Autodesk Inventor part; units mm, degrees
ref_plane "YZ Plane" through (0, 0, 0) normal (1, 0, 0) x (0, 1, 0)
ref_plane "XZ Plane" through (0, 0, 0) normal (0, 1, 0) x (-1, 0, 0)
ref_plane "XY Plane" through (0, 0, 0) normal (0, 0, 1) x (1, 0, 0)
sketch "Sketch1" plane through (0, 0, 0) normal (0, 0, 1) x (1, 0, 0)
  line L0 (-35.5, 13.25) -> (35.5, 13.25)
  line L1 (35.5, 13.25) -> (35.5, -13.25)
  line L2 (35.5, -13.25) -> (-35.5, -13.25)
  line L3 (-35.5, -13.25) -> (-35.5, 13.25)
  line L4 (-34.3, 12.05) -> (34.3, 12.05)
  line L5 (34.3, 12.05) -> (34.3, -12.05)
  line L6 (34.3, -12.05) -> (-34.3, -12.05)
  line L7 (-34.3, -12.05) -> (-34.3, 12.05)
  point P0 (0, 0)
  dimension "d0" = 71
  dimension "d1" = 26.5
  dimension "d2" = 35.5
  dimension "d3" = 13.25
  dimension "d4" = 1.2
  dimension "d5" = 1.2
  dimension "d6" = 1.2
  dimension "d7" = 1.2
extrude "Extrusion1" add sketch "Sketch1" along normal blind 100
fillet "Fillet1" radius 2 4 edges at (-34.3, 12.05, 50) (34.3, 12.05, 50) (34.3, -12.05, 50) (-34.3, -12.05, 50)
fillet "Fillet2" radius 3.25 4 edges at (-35.5, 13.25, 50) (-35.5, -13.25, 50) (35.5, -13.25, 50) (35.5, 13.25, 50)
sketch "Sketch2" plane through (0, 0, 100) normal (0, 0, 1) x (1, 0, 0)
  line L0 (-34.3, -10.05) -> (-34.3, 10.05)
  line L1 (-34.3, -7.9) -> (-31.3, -7.9)
  line L2 (-31.3, -7.9) -> (-31.3, -9.4)
  line L3 (-31.3, -9.4) -> (-34.3, -9.4)
  line L4 (-34.3, -9.4) -> (-34.3, -7.9)
  line L5 (34.3, 10.05) -> (34.3, -10.05)
  line L6 (34.3, -7.9) -> (31.3, -7.9)
  line L7 (31.3, -7.9) -> (31.3, -9.4)
  line L8 (31.3, -9.4) -> (34.3, -9.4)
  line L9 (34.3, -9.4) -> (34.3, -7.9)
  line L10 (-32.25, -13.25) -> (32.25, -13.25)
  line L11 (-34.3, -5.9) -> (-31.3, -5.9)
  line L12 (-31.3, -5.9) -> (-31.3, -4.4)
  line L13 (-31.3, -4.4) -> (-34.3, -4.4)
  line L14 (-34.3, -4.4) -> (-34.3, -5.9)
  line L15 (31.3, -5.9) -> (34.3, -5.9)
  line L16 (34.3, -5.9) -> (34.3, -4.4)
  line L17 (34.3, -4.4) -> (31.3, -4.4)
  line L18 (31.3, -4.4) -> (31.3, -5.9)
  point P0 (0, 0)
  dimension "d12" = 3.85
  dimension "d13" = 1.5
  dimension "d14" = 3
  dimension "d15" = 3
  dimension "d16" = 1.5
  dimension "d17" = 2
extrude "Extrusion2" add sketch "Sketch2" against normal blind 100
fillet "Fillet3" radius 1 4 edges at (-34.3, -4.4, 50) (-34.3, -9.4, 50) (34.3, -9.4, 50) (34.3, -4.4, 50)
sketch "Sketch3" plane through (0, 0, 100) normal (0, 0, 1) x (1, 0, 0)
  line L0 (32.25, 13.25) -> (-32.25, 13.25)
  line L1 (-35.5, 10) -> (-35.5, -10)
  line L2 (-32.25, -13.25) -> (32.25, -13.25)
  line L3 (35.5, -10) -> (35.5, 10)
  circle A0 centre (-32.5, 10.25) radius 2.25
  circle A1 centre (-32.5, -10.25) radius 2.25
  circle A2 centre (32.5, -10.25) radius 2.25
  circle A3 centre (32.5, 10.25) radius 2.25
  point P0 (0, 0)
  dimension "d21" = 3
  dimension "d22" = 3
  dimension "d23" = 3
  dimension "d24" = 3
  dimension "d25" = 3
  dimension "d26" = 3
  dimension "d27" = 3
  dimension "d28" = 3
  dimension "d29" = 4.5
  dimension "d30" = 4.5
  dimension "d31" = 4.5
  dimension "d32" = 4.5
extrude "Extrusion3" add sketch "Sketch3" against normal blind 100
sketch "Sketch4" plane through (0, 0, 100) normal (0, 0, 1) x (1, 0, 0)
  arc A0 (-34.3, 8.9) -> (-31.15, 12.05) centre (-32.5, 10.25) ccw
  arc A1 (31.15, 12.05) -> (34.3, 8.9) centre (32.5, 10.25) ccw
  arc A2 (31.3, -8.3467) -> (31.15, -12.05) centre (32.5, -10.25) ccw
  arc A3 (-31.15, -12.05) -> (-31.3, -8.3467) centre (-32.5, -10.25) ccw
  circle A4 centre (-32.5, 10.25) radius 1.25
  circle A5 centre (-32.5, -10.25) radius 1.25
  circle A6 centre (32.5, 10.25) radius 1.25
  circle A7 centre (32.5, -10.25) radius 1.25
  point P0 (0, 0)
  dimension "d35" = 2.5
  dimension "d36" = 2.5
  dimension "d37" = 2.5
  dimension "d38" = 2.5
extrude "Extrusion4" cut sketch "Sketch4" against normal blind 100
sketch "Sketch6" plane through (0, 0, 100) normal (0, 0, 1) x (1, 0, 0)
  line L0 (34.3, -5.9) -> (34.3, -7.9)
  line L1 (-34.3, -7.9) -> (-34.3, -5.9)
  line L2 (-31.3, -7.9) -> (-34.3, -7.9)
  line L3 (-31.3, -7.9) -> (-31.5, -7.9)
  line L4 (-31.5, -7.9) -> (-31.5, -9.4)
  line L5 (-31.5, -9.4) -> (-31.3, -9.4)
  line L6 (-31.3, -9.4) -> (-31.3, -7.9)
  line L7 (-31.3, -5.9) -> (-31.3, -4.4)
  line L8 (-31.3, -4.4) -> (-31.5, -4.4)
  line L9 (-31.5, -4.4) -> (-31.5, -5.9)
  line L10 (-31.5, -5.9) -> (-31.3, -5.9)
  line L11 (-31.3, -5.9) -> (-31.3, -4.4)
  line L12 (31.3, -4.4) -> (31.5, -4.4)
  line L13 (31.5, -4.4) -> (31.5, -5.9)
  line L14 (31.5, -5.9) -> (31.3, -5.9)
  line L15 (31.3, -5.9) -> (31.3, -4.4)
  line L16 (31.3, -7.9) -> (31.5, -7.9)
  line L17 (31.5, -7.9) -> (31.5, -9.4)
  line L18 (31.5, -9.4) -> (31.3, -9.4)
  line L19 (31.3, -9.4) -> (31.3, -7.9)
  line L20 (-31.3, -5.9) -> (-34.3, -5.9)
  line L21 (-34.3, -5.9) -> (-32.5, -5.9)
  line L22 (-32.5, -5.9) -> (-32.5, -7.9)
  line L23 (-32.5, -7.9) -> (-34.3, -7.9)
  line L24 (-34.3, -7.9) -> (-34.3, -5.9)
  line L25 (34.3, -5.9) -> (31.3, -5.9)
  line L26 (31.3, -7.9) -> (34.3, -7.9)
  line L27 (34.3, -5.9) -> (32.5, -5.9)
  line L28 (32.5, -5.9) -> (32.5, -7.9)
  line L29 (32.5, -7.9) -> (34.3, -7.9)
  line L30 (34.3, -7.9) -> (34.3, -5.9)
  point P0 (0, 0)
  point P1 (32.5, -5.9)
  point P2 (-31.5, -5.9)
  dimension "d46" = 68.6
  dimension "d47" = 65
  dimension "d48" = 1.8
  dimension "d49" = 1.8
  dimension "d50" = 1
  dimension "d51" = 1.5
  dimension "d52" = 1
extrude "Extrusion6" add sketch "Sketch6" against normal blind 100 contours L0 L26 L28 L25 | L1 L20 L22 L2
sketch "Sketch7" plane through (0, 0, 100) normal (0, 0, 1) x (1, 0, 0)
  line L0 (-32.25, -13.25) -> (32.25, -13.25)
  line L1 (32.25, 13.25) -> (-32.25, 13.25)
  line L2 (35.5, -10) -> (35.5, 10)
  line L3 (-35.5, 10) -> (-35.5, -10)
  line L4 (-34.1, -5.9) -> (34.1, -5.9)
  line L5 (34.1, -5.9) -> (34.1, -7.9)
  line L6 (34.1, -7.9) -> (-34.1, -7.9)
  line L7 (-34.1, -7.9) -> (-34.1, -5.9)
  line L8 (-32.5, -5.9) -> (-31.3, -5.9)
  line L9 (-31.3, -7.9) -> (-32.5, -7.9)
  line L10 (-32.5, -7.9) -> (-32.5, -5.9)
  line L11 (32.5, -5.9) -> (32.5, -7.9)
  point P0 (0, 0)
  point P1 (35.5, 4.9)
  point P2 (-29.5, -6.05)
  point P3 (-29.5, -7.9)
  dimension "d55" = 26.5
  dimension "d56" = 71
  dimension "d57" = 68.2
  dimension "d58" = 1.6
  dimension "d59" = 1.6
extrude "Extrusion7" cut sketch "Sketch7" against normal blind 200
fillet "Fillet4" radius 1 6 edges at (-34.3, 8.9, 50) (-31.15, 12.05, 50) (31.15, 12.05, 50) (34.3, 8.9, 50) (31.15, -12.05, 50) (-31.15, -12.05, 50)
properties part number "case"
Source: CAD feature listing. Evaluate the final solid. Frame: model axes, mm. A direction names the side the tool comes from. Coordinates: 2 decimals unless noted, no trailing zeros. Order: outer loops, then holes, each group sorted by start corner. A loop starts at its lowest first (then second) coordinate and runs counter-clockwise, first axis right, second up. Notation, with made-up numbers: M -6.5,0.5 L -2.5,0.5 A18 cw -2.5,34.5 Z; hole C 58.5,73.5 d7. An arc over 180 degrees is marked long. Write each question's results on one line, items separated by ' | '. Start each with the question number.
Item 1: Cut plane C-C (z = 60). Count the separate pieces of the cut face and the enclosed holes in it, and give its area (3 significant figures).
Item 2: Line query: probe 1 along Y at (x, z) = (-32.5, 43); probe 2 along Y at (x, z) = (20, 20); probe 3 along X at (y, z) = (-3.5, 78). Output: solid intervals per line, ascending.
Item 3: Draft query along X for faces 3 (the face through (-5, 13, 0)), 4 (the face through (-34.573, -12.273, 50.7)), 5 (the face through (-31.828, 11.304, 50.7)). Return one class per face: pulls with the +X half, pulls with the -X half, needs draft (parallel to the pull), parting line crosses it, or undercut.
Item 4: Cut plane A-A (y = -1). Return loops of the section in (x, z).
Item 5: Set-up query: faces 1 (the face through (0, -12.05, 49)), 2 (the face through (-5, 13, 100)). Return all of +Z, -Z, +X, -X, +Y, -Y with unobstructed straight access to the full face (end or side cutting, diameter ignored); none if empty.
Item 6: Cut plane B-B (x = -14). Return loops of the section in (y, z).
Item 7: First-contact query: pin 1 Ø5 at (x, y) = (-2, 8.5) entering from +Z. Flat tip, straight axial feed; report the tip coordinate or a pass-through.
Checked values:
1) separate pieces: 1 | enclosed holes: 5 | area: 272 mm2
2) probe 1: y = -13.24 to -11.5, -9 to -7.9, -5.9 to -4.4, 8 to 9, 11.5 to 13.24 | probe 2: y = -13.25 to -12.05, 12.05 to 13.25 | probe 3: x = -35.5 to -34.29, 34.29 to 35.5
3) face 3: needs draft | face 4: pulls with the -X half | face 5: undercut
4) outline: M -35.5,0 L -34.3,0 L -34.3,100 L -35.5,100 Z; M 34.3,0 L 35.5,0 L 35.5,100 L 34.3,100 Z
5) face 1: +Z, -Z | face 2: +Z, +X, -X, +Y, -Y
6) outline: M -13.25,0 L -12.05,0 L -12.05,100 L -13.25,100 Z; M 12.05,0 L 13.25,0 L 13.25,100 L 12.05,100 Z
7) pin 1: passes through
